Autodesk Inventor part; units mm, degrees
ref_plane "YZ Plane" through (0, 0, 0) normal (1, 0, 0) x (0, 1, 0)
ref_plane "XZ Plane" through (0, 0, 0) normal (0, 1, 0) x (-1, 0, 0)
ref_plane "XY Plane" through (0, 0, 0) normal (0, 0, 1) x (1, 0, 0)
sketch "Sketch1" plane through (0, 0, 0) normal (0, 1, 0) x (-1, 0, 0)
  line L0 (15.9, 7.9) -> (-15.9, 7.9)
  line L1 (-15.9, 7.9) -> (-15.9, -7.9)
  line L2 (-15.9, -7.9) -> (15.9, -7.9)
  line L3 (15.9, -7.9) -> (15.9, 7.9)
  line L4 (15.9, 7.9) -> (-15.9, -7.9) construction
  line L5 (-15.9, 7.9) -> (15.9, -7.9) construction
  point P0 (0, 0)
  dimension "d0" = 31.8
  dimension "d1" = 15.8
extrude "Extrusion1" add sketch "Sketch1" along normal blind 9.6
sketch "Sketch2" plane through (0, 0, 0) normal (0, -1, 0) x (1, 0, 0)
  line L0 (-14.7, -6.7) -> (14.7, -6.7)
  line L1 (14.7, -6.7) -> (14.7, 6.7)
  line L2 (14.7, 6.7) -> (-14.7, 6.7)
  line L3 (-14.7, 6.7) -> (-14.7, -6.7)
  line L4 (-14.7, -6.7) -> (14.7, 6.7) construction
  line L5 (14.7, -6.7) -> (-14.7, 6.7) construction
  line L6 (-15.9, 7.9) -> (15.9, 7.9)
  line L7 (15.9, 7.9) -> (15.9, -7.9)
  point P0 (0, 0)
  dimension "d4" = 1.2
  dimension "d5" = 1.2
extrude "Extrusion2" cut sketch "Sketch2" against normal blind 8.6
sketch "Sketch3" plane through (0, 9.6, 0) normal (0, 1, 0) x (1, 0, 0)
  circle A0 centre (12, 4) radius 2.4
  line L0 (15.9, -7.9) -> (15.9, 7.9)
  point P0 (0, 0)
  dimension "d8" = 4.8
  dimension "d9" = 3.9
  dimension "d10" = 4
extrude "Extrusion3" add sketch "Sketch3" along normal blind 1.8
sketch "Sketch4" plane through (0, 8.6, 0) normal (0, -1, 0) x (1, 0, 0)
  circle A0 centre (12, -4) radius 2.4
  point P0 (0, 0)
hole "Hole1" at (12, 8.6, -4) direction (0, 1, 0) diameter 2.6 depth 1.7
pattern_linear "Rectangular Pattern1" count 4 spacing 8 along (-1, 0, 0) count 2 spacing 8 along (0, 0, 1) of "Extrusion3"
pattern_linear "Rectangular Pattern2" count 4 spacing 8 along (-1, 0, 0) count 2 spacing 8 along (0, 0, 1) of "Hole1"
sketch "Sketch5" plane through (0, 8.6, 0) normal (0, -1, 0) x (1, 0, 0)
  circle A0 centre (0, 0) radius 3.255
  circle A1 centre (0, 0) radius 2.4
  dimension "d32" = 6.51
  dimension "d33" = 4.8
extrude "Extrusion4" add sketch "Sketch5" along normal up to surface (8.6 mm away)
pattern_linear "Rectangular Pattern3" count 2 spacing 8 along (-1, 0, 0) of "Extrusion4"
pattern_linear "Rectangular Pattern4" count 2 spacing 8 along (1, 0, 0) of "Extrusion4"
sketch "Sketch6" plane through (0, 8.6, 0) normal (0, -1, 0) x (1, 0, 0)
  circle A0 centre (0, 0) radius 3.255
  line L0 (-14.7, 6.7) -> (14.7, 6.7)
  line L1 (-0.4, 6.7) -> (-0.4, 3.2303)
  line L2 (0.4, 6.7) -> (0.4, 3.2303)
  dimension "d42" = 0.4
  dimension "d43" = 0.4
extrude "Extrusion5" add sketch "Sketch6" along normal blind 6.3 contours A0 L1 L0 L2
mirror "Mirror1" about plane through (0, 0, 0) normal (0, 0, 1) of "Extrusion5"
sketch "Sketch7" plane through (0, 0, 0) normal (0, -1, 0) x (1, 0, 0)
  line L0 (14.7, -6.7) -> (-14.7, -6.7)
  line L1 (-12.3, -6.9) -> (-11.7, -6.9)
  line L2 (-11.7, -6.9) -> (-11.7, -6.5)
  line L3 (-11.7, -6.5) -> (-12.3, -6.5)
  line L4 (-12.3, -6.5) -> (-12.3, -6.9)
  line L5 (-12.3, -6.9) -> (-11.7, -6.5) construction
  line L6 (-11.7, -6.9) -> (-12.3, -6.5) construction
  line L7 (-15.9, -7.9) -> (-15.9, 7.9)
  point P0 (0, 0)
  point P1 (-12, -6.7)
  dimension "d46" = 3.9
  dimension "d47" = 0.6
  dimension "d48" = 0.4
extrude "Extrusion6" add sketch "Sketch7" against normal up to surface (8.6 mm away)
pattern_linear "Rectangular Pattern5" count 4 spacing 8 along (1, 0, 0) of "Extrusion6"
sketch "Sketch8" plane through (0, 8.6, 0) normal (0, -1, 0) x (1, 0, 0)
  line L0 (-14.7, 6.7) -> (14.7, 6.7)
  line L1 (12.3, 6.8) -> (11.7, 6.8)
  line L2 (11.7, 6.8) -> (11.7, 6.6)
  line L3 (11.7, 6.6) -> (12.3, 6.6)
  line L4 (12.3, 6.6) -> (12.3, 6.8)
  line L5 (0.4, 6.7) -> (14.7, 6.7)
  line L6 (12.3, 6.8) -> (11.7, 6.6) construction
  line L7 (11.7, 6.8) -> (12.3, 6.6) construction
  line L8 (15.9, 7.9) -> (15.9, -7.9)
  point P0 (0, 0)
  point P1 (12, 6.7)
  dimension "d54" = 3.9
  dimension "d55" = 0.6
  dimension "d56" = 0.2
extrude "Extrusion7" add sketch "Sketch8" along normal up to surface (8.6 mm away)
pattern_linear "Rectangular Pattern6" count 4 spacing 8 along (-1, 0, 0) of "Extrusion7"
sketch "Sketch9" plane through (0, 8.6, 0) normal (0, -1, 0) x (1, 0, 0)
  line L0 (-14.5, -3.7) -> (-14.9, -3.7)
  line L1 (-14.9, -3.7) -> (-14.9, -4.3)
  line L2 (-14.9, -4.3) -> (-14.5, -4.3)
  line L3 (-14.5, -4.3) -> (-14.5, -3.7)
  line L4 (-14.7, -6.7) -> (-14.7, 6.7)
  line L5 (-14.5, -3.7) -> (-14.9, -4.3) construction
  line L6 (-14.9, -3.7) -> (-14.5, -4.3) construction
  point P0 (0, 0)
  point P1 (-14.7, -4)
  dimension "d62" = 0.6
  dimension "d63" = 0.4
  dimension "d64" = 4
extrude "Extrusion8" add sketch "Sketch9" along normal up to surface (8.6 mm away)
pattern_linear "Rectangular Pattern7" count 2 spacing 8 along (0, 0, 1) of "Extrusion8"
sketch "Sketch10" plane through (0, 8.6, 0) normal (0, -1, 0) x (1, 0, 0)
  line L0 (14.7, 6.7) -> (14.7, -6.7)
  line L1 (14.9, -3.7) -> (14.5, -3.7)
  line L2 (14.5, -3.7) -> (14.5, -4.3)
  line L3 (14.5, -4.3) -> (14.9, -4.3)
  line L4 (14.9, -4.3) -> (14.9, -3.7)
  line L5 (14.7, 6.7) -> (14.7, -6.7)
  line L6 (14.9, -3.7) -> (14.5, -4.3) construction
  line L7 (14.5, -3.7) -> (14.9, -4.3) construction
  point P0 (0, 0)
  point P1 (14.7, -4)
  dimension "d70" = 4
  dimension "d71" = 0.6
  dimension "d72" = 0.4
extrude "Extrusion9" add sketch "Sketch10" along normal up to surface (8.6 mm away)
mirror "Mirror2" about plane through (0, 0, 0) normal (0, 0, 1) of "Extrusion9"
sketch "Sketch11" plane through (0, 0, 0) normal (0, 1, 0) x (-1, 0, 0)
  point P0 (0, 0)
properties part number "Lego Brick"
Geometry check sheet. Reference: the model listing, model coordinates, mm. A direction names the side the tool comes from. Round coordinates to 2 decimals unless told otherwise and drop trailing zeros. Loops run counter-clockwise (first coordinate to the right, second up) from the corner with the lowest first, then second, coordinate; pieces in that order, holes last. Notation, with made-up numbers: (-8, -5.5) - (38, -5.5) arc R20 ccw to (38, 13.5) - close; hole circle Ø9 at (-3, 47.5). An arc over 180 degrees is marked (long way). Answer as CSV lines item,"result".
(1) Depth check by flat-ended pin: pin 1 Ø3 at (x, z) = (9.5, 3.5) entering from +Y; pin 2 Ø1.5 at (x, z) = (-0.5, -5) entering from +Y; pin 3 Ø3 at (x, z) = (12.5, -4) entering from -Y; pin 4 Ø1.3 at (x, z) = (-12, -3.5) entering from -Y. Enter the tip coordinate at first touch or a pass-through.
Output values:
pin 1,"stops at y = 11.4"
pin 2,"stops at y = 9.6"
pin 3,"stops at y = 8.6"
pin 4,"stops at y = 10.3"
(2) Cross-section at A-A, the plane x = 0. Enter the section's corners in (y, z) (3 decimals), and give its area (3 significant figures).
Output values:
outline,"(0, -7.9) - (9.6, -7.9) - (9.6, 7.9) - (0, 7.9) - (0, 6.7) - (2.3, 6.7) - (2.3, 3.255) - (0, 3.255) - (0, 2.4) - (8.6, 2.4) - (8.6, -2.4) - (0, -2.4) - (0, -3.255) - (2.3, -3.255) - (2.3, -6.7) - (0, -6.7) - close"
area,"94.6 mm²"
(3) Cross-section at C-C, the plane y = 1. Give the number of separate pieces and of enclosed holes in the cut face, and give its area (3 significant figures).
Output values:
separate pieces,"4"
enclosed holes,"4"
area,"155 mm²"
(4) Release check for a two-part mould opening along Z. For faces 1 (the face through (-12, 11.4, -4)), 2 (the face through (14.7, 4, -6)), 3 (the face through (0, 5, -7.9)) record: released by +Z, released by -Z, zero draft, split by the parting line, or undercut.
Output values:
face 1,"zero draft"
face 2,"undercut"
face 3,"released by -Z"
(5) Material ranges on line 1 along X through (y, z) = (3.5, 5); line 2 along X through (y, z) = (7, -4.25); line 3 along Z through (x, y) = (-8, 6) (3 decimals), recorded low to high.
Output values:
line 1,"x = -15.9 to -14.7, -0.4 to 0.4, 14.7 to 15.9"
line 2,"x = -15.9 to -14.5, -0.4 to 0.4, 14.5 to 15.9"
line 3,"z = -7.9 to -6.7, -3.255 to -2.4, 2.4 to 3.255, 6.7 to 7.9"
(6) Set-up check for faces 4 (the face through (-2.847, 9.462, -4.6)), 5 (the face through (-14.398, 10.487, -3.894)), 6 (the face through (4, 11.4, -4)): record each of +Z, -Z, +X, -X, +Y, -Y from which the full face is reachable in a straight line by a thin tool's end or side.
Output values:
face 4,"-Y"
face 5,"+Y"
face 6,"+Z, -Z, +X, -X, +Y"
